Geometry check sheet. Reference: the model listing, model coordinates, mm. A direction names the side the tool comes from. Give positions to 0.01 mm unless a question says otherwise; leave off trailing zeros. Loops run counter-clockwise (first coordinate to the right, second up) from the corner with the lowest first, then second, coordinate; pieces in that order, holes last. Notation, with made-up numbers: (32.5, -5) - (86.5, -5) arc R21 ccw to (86.5, 2) - close; hole circle Ø8 at (54, 69.25). An arc over 180 degrees is marked (long way). Use a Markdown table: item, result. Add a question column.
1. Set-up check for faces 4 (the flat face through (5, 20.5, 6)), 5 (the cylindrical face through (9.699, 21.514, 8.715)), 6 (the cylindrical face through (1.699, 25.035, 8.715)), 7 (the flat face through (0, 25, 3)), 8 (the flat face through (5, 40, 3)): record each of +Z, -Z, +X, -X, +Y, -Y from which the full face is reachable in a straight line by a thin tool's end or side.
2. Material ranges on L1, parallel to Z at x = 7, y = 28.55; L2, parallel to Y at x = 5.25, z = 4; L3, parallel to X at y = 29, z = 7.75, recorded low to high.
3. Cross-section at B-B on z = 7. Enter the section's corners in (x, y).
4. Cross-section at D-D on z = 0.5. Enter the section's corners in (x, y), and give its area (3 significant figures).
5. Depth check by flat-ended pin: P1, Ø3.5, axis at x = 7, z = 7, coming from the -Y side; P2, Ø2.5, axis at x = 6.5, z = 7.5, coming from the +Y side; P3, Ø3, axis at x = 6.5, y = 41.5, coming from the +Z side. Enter the tip coordinate at first touch or a pass-through.
6. Draft check along Y on faces 1 (the flat face through (2, 25, 5)), 2 (the flat face through (9.5, 24.7, 0.5)), 3 (the flat face through (5, 29.5, 6)). Enter one of: pulls with the +Y half, pulls with the -Y half, needs draft (parallel to the pull), parting line crosses it, or undercut.
7. Cross-section at C-C on y = 43. Enter the section's corners in (x, z).
8. Cross-section at A-A on x = 7. Enter the section's corners in (y, z), and give its area (3 significant figures).
from build123d import *

# Parameters (mm, degrees)
SKETCH1_W           = 10
SKETCH1_H           = 50
BOSS_EXTRUDE1_DEPTH = 3
CHAMFER1_SIZE       = 1
SKETCH2_W           = 10
SKETCH2_H           = 2
BOSS_EXTRUDE2_DEPTH = 6
SKETCH3_R           = 1.5
CUT_EXTRUDE1_DEPTH  = 10
FILLET1_R           = 1
FILLET2_R           = 1
SKETCH4_W           = 6
SKETCH4_H           = 5
BOSS_EXTRUDE3_DEPTH = 2
FILLET3_R           = 1


with BuildPart() as part:
    # Sketch1 → Boss-Extrude1 (new body)
    with BuildSketch(Plane.XY):
        with Locations((5, 25)):
            Rectangle(SKETCH1_W, SKETCH1_H)
    extrude(amount=BOSS_EXTRUDE1_DEPTH)

    # Chamfer1
    chamfer1_edges = [part.edges().sort_by_distance(p)[0] for p in [
        (5, 50, 0),
        (10, 25, 0),
        (5, 0, 0),
        (0, 25, 0),
    ]]
    chamfer(chamfer1_edges, length=CHAMFER1_SIZE)

    # Sketch2 → Boss-Extrude2 (add)
    with BuildSketch(Plane.XY.offset(3)):
        with Locations((5, 28.5)):
            Rectangle(SKETCH2_W, SKETCH2_H)
        with Locations((5, 21.5)):
            Rectangle(SKETCH2_W, SKETCH2_H)
    extrude(amount=BOSS_EXTRUDE2_DEPTH)

    # Sketch3 → Cut-Extrude1 (cut)
    with BuildSketch(Plane.XZ.offset(-20.5)):
        with Locations((7, 7)):
            Circle(SKETCH3_R)
    extrude(amount=-CUT_EXTRUDE1_DEPTH, mode=Mode.SUBTRACT)

    # Fillet1
    fillet1_edges = [part.edges().sort_by_distance(p)[0] for p in [
        (10, 28.5, 9),
        (10, 21.5, 9),
    ]]
    fillet(fillet1_edges, radius=FILLET1_R)

    # Fillet2
    fillet2_edges = [part.edges().sort_by_distance(p)[0] for p in [
        (5, 29.5, 3),
        (5, 20.5, 3),
    ]]
    fillet(fillet2_edges, radius=FILLET2_R)

    # Sketch4 → Boss-Extrude3 (add)
    with BuildSketch(Plane.ZY):
        with Locations((6, 25)):
            Rectangle(SKETCH4_W, SKETCH4_H)
    extrude(amount=-BOSS_EXTRUDE3_DEPTH)

    # Fillet3
    fillet3_edges = [part.edges().sort_by_distance(p)[0] for p in [
        (2, 25, 9),
    ]]
    fillet(fillet3_edges, radius=FILLET3_R)


solid = part.part
Values found:
| question | item | result |
|---|---|---|
| 1 | face 4 | +Z, +X, -X, -Y |
| 1 | face 5 | +Z, +X, +Y, -Y |
| 1 | face 6 | +Z, +X |
| 1 | face 7 | +Z, -Z, -X, +Y, -Y |
| 1 | face 8 | +Z, +X, -X, +Y |
| 2 | L1 | z = 0 to 5.5, 8.5 to 9 |
| 2 | L2 | y = 20.5 to 22.5, 27.5 to 29.5 |
| 2 | L3 | x = 0 to 5.7, 8.3 to 10 |
| 3 | outline | (0, 20.5) - (5.5, 20.5) - (5.5, 22.5) - (2, 22.5) - (2, 27.5) - (5.5, 27.5) - (5.5, 29.5) - (0, 29.5) - close; (8.5, 20.5) - (10, 20.5) - (10, 22.5) - (8.5, 22.5) - close; (8.5, 27.5) - (10, 27.5) - (10, 29.5) - (8.5, 29.5) - close |
| 4 | outline | (0.5, 0.5) - (9.5, 0.5) - (9.5, 49.5) - (0.5, 49.5) - close |
| 4 | area | 441 mm2 |
| 5 | P1 | stops at y = 20.5 |
| 5 | P2 | stops at y = 29.5 |
| 5 | P3 | stops at z = 3 |
| 6 | face 1 | undercut |
| 6 | face 2 | needs draft |
| 6 | face 3 | pulls with the +Y half |
| 7 | outline | (0, 1) - (1, 0) - (9, 0) - (10, 1) - (10, 3) - (0, 3) - close |
| 8 | outline | (0, 1) - (1, 0) - (49, 0) - (50, 1) - (50, 3) - (30.5, 3) arc R1 cw to (29.5, 4) - (29.5, 5.5) - (27.5, 5.5) - (27.5, 3) - (22.5, 3) - (22.5, 5.5) - (20.5, 5.5) - (20.5, 4) arc R1 cw to (19.5, 3) - (0, 3) - close; (20.5, 8.5) - (22.5, 8.5) - (22.5, 9) - (20.5, 9) - close; (27.5, 8.5) - (29.5, 8.5) - (29.5, 9) - (27.5, 9) - close |
| 8 | area | 161 mm2 |
